Autodesk Inventor part; units mm, degrees
ref_plane "YZ Plane" through (0, 0, 0) normal (1, 0, 0) x (0, 1, 0)
ref_plane "XZ Plane" through (0, 0, 0) normal (0, 1, 0) x (-1, 0, 0)
ref_plane "XY Plane" through (0, 0, 0) normal (0, 0, 1) x (1, 0, 0)
sketch "Sketch1" plane through (0, 0, 0) normal (0, 0, 1) x (1, 0, 0)
  circle A0 centre (0, 0) radius 9
  circle A1 centre (0, 0) radius 1.5
  dimension "d0" = 18
  dimension "d1" = 3
extrude "Extrusion1" add sketch "Sketch1" along normal blind 4.6
sketch "Sketch2" plane through (0, 0, 4.6) normal (0, 0, 1) x (1, 0, 0)
  circle A0 centre (7, 0) radius 0.75
  point P0 (0, 0)
  dimension "d4" = 7
  dimension "d5" = 1.5
extrude "Extrusion2" cut sketch "Sketch2" against normal blind 5
pattern_circular "Circular Pattern1" count 12 over 360 about axis through (0, 0, 0) along (0, 0, 1) of "Extrusion2"
properties part number "herkulex spinner"
For this review, take the finished solid that the model builds, in its own axes (mm). Coordinates: 2 decimals unless noted, no trailing zeros. Loops run counter-clockwise (first coordinate to the right, second up) from the corner with the lowest first, then second, coordinate; pieces in that order, holes last. Notation, with made-up numbers: (37, -22) - (49, -22) arc R35 ccw to (49, 12) - close; hole circle Ø10 at (-2.75, 89.5). An arc over 180 degrees is marked (long way). Use one line per item in the form item = value. Start each with the question number.
1) Take a section at D-D (y = -3.5). State the section outline as (x, z) points, plus the area to 3 significant figures.
2) Take a section at B-B (y = -0.25). State the section outline as (x, z) points, plus the area to 3 significant figures.
3) To check wall thickness, follow probe 1 along Y at (x, z) = (6.5, 1.65); probe 2 along X at (y, z) = (-5.5, 1.45); probe 3 along Y at (x, z) = (-6, 1.6). State the ranges of each line that lie inside material, in increasing order. Write a range as from..to.
4) Draft analysis for pull direction Y (two halves, no side actions). For faces 1 (the face through (0, -2, 0)), 2 (the face through (0.03, -6.25, 2.33)), 3 (the face through (-1.172, -8.923, 2.268)), 4 (the face through (3.598, -6.806, 2.332)), state which applies: released by +Y, released by -Y, zero draft, split by the parting line, or undercut.
5) Take a section at C-C (z = 0.9). State how many separate pieces and enclosed holes the cut face has, plus the area to 3 significant figures.
6) For pin 1 (1 mm diameter, centred on x = 5, z = 1.5, fed in from -Y), flat-tipped, find the tip position at first contact; note if it passes through.
7) Take a section at A-A (x = 0). State the section outline as (y, z) points.
From the geometry:
q1.outline = (-8.29, 0) - (-6.81, 0) - (-6.81, 4.6) - (-8.29, 4.6) - close; (-5.31, 0) - (5.31, 0) - (5.31, 4.6) - (-5.31, 4.6) - close; (6.81, 0) - (8.29, 0) - (8.29, 4.6) - (6.81, 4.6) - close
q1.area = 62.5 mm2
q2.outline = (-9, 0) - (-7.71, 0) - (-7.71, 4.6) - (-9, 4.6) - close; (-6.29, 0) - (-1.48, 0) - (-1.48, 4.6) - (-6.29, 4.6) - close; (1.48, 0) - (6.29, 0) - (6.29, 4.6) - (1.48, 4.6) - close; (7.71, 0) - (9, 0) - (9, 4.6) - (7.71, 4.6) - close
q2.area = 56.2 mm2
q3.probe_1 = -6.22..-4.11, -2.89..-0.56, 0.56..2.89, 4.11..6.22
q3.probe_2 = -7.12..-4, -3..3, 4..7.12
q3.probe_3 = -6.71..-4.25, -2.75..2.75, 4.25..6.71
q4.face_1 = zero draft
q4.face_2 = undercut
q4.face_3 = split by the parting line
q4.face_4 = undercut
q5.separate_pieces = 1
q5.enclosed_holes = 13
q5.area = 226 mm2
q6.pin_1 = -7.79
q7.outline = (-9, 0) - (-7.75, 0) - (-7.75, 4.6) - (-9, 4.6) - close; (-6.25, 0) - (-1.5, 0) - (-1.5, 4.6) - (-6.25, 4.6) - close; (1.5, 0) - (6.25, 0) - (6.25, 4.6) - (1.5, 4.6) - close; (7.75, 0) - (9, 0) - (9, 4.6) - (7.75, 4.6) - close
